Can you work these out from the model? Positions are in its coordinate system, mm. Face numbers are marked on the shaded views. A direction names the side the tool comes from. Coordinates: 2 decimals unless noted, no trailing zeros. Order: outer loops, then holes, each group sorted by start corner. A loop starts at its lowest first (then second) coordinate and runs counter-clockwise, first axis right, second up. Notation, with made-up numbers: (27.25, -7.75) -> (66.25, -7.75) arc R10 cw to (66.25, -0.75) -> close; hole circle Ø9 at (11.5, 70). An arc over 180 degrees is marked (long way). Return JSON: item names as keys, results as strings. Group by question number.
1) If we section it at B-B, the plane z = -7.5: Please give me the cut outline in (x, y).
2) Thinking about a two-plate mould opening in Z: for the marked faces 3, 4 and 5, which applies, +Z half, -Z half, draft (parallel to the pull), parting line (faces both ways), or undercut?
3) If I drill on probe 1 along Z at (x, y) = (0.5, -4); probe 2 along Z at (x, y) = (6.5, -11.5); probe 3 along Z at (x, y) = (-8.89, -7) (3 decimals), over which ranges is the centre line in solid material (lowest first)? Write a range as from..to.
4) For pin 1 (6.5 mm diameter, centred on y = -11.5, z = -25.5, fed in from +X); pin 2 (5 mm diameter, centred on x = 10, z = -53, fed in from +Y); pin 3 (9 mm diameter, centred on y = -11, z = -28.5, fed in from -X), each with a flat end and sliding along its axis, tell me the tip position at first contact or that it passes through.
5) If we section it at A-A, the plane z = -66.04: Please give me the cut outline in (x, y) (3 decimals).
6) If we section it at C-C, the plane x = 0: Please give me the cut outline in (y, z), then the cut area to 3 significant figures.
7) If we section it at D-D, the plane y = -3.5: State how many separate pieces and enclosed holes the cut face has, then the cut area to 3 significant figures.
8) For the marked faces 1 and 2, which set-ups out of +Z, -Z, +X, -X, +Y, -Y let a thin tool reach every point of the face, with its end or its side?
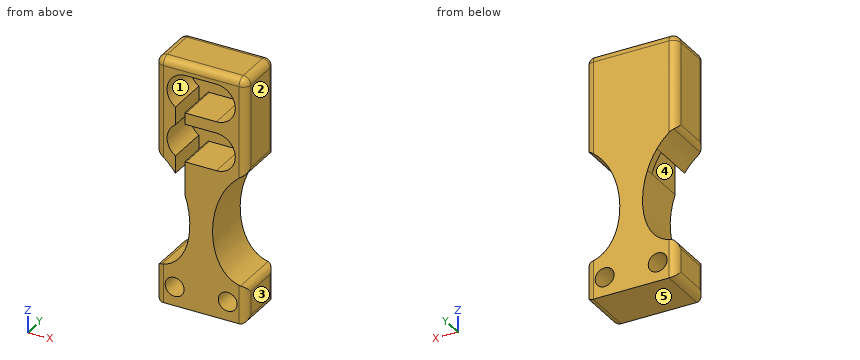
from build123d import *

# Parameters (mm, degrees)
F0_R     = 3.175
F1_DEPTH = 16.51
F2_DEPTH = 2.54
F3_R     = 2.54


# Not quite as in the source:
# - a feature names something its author has since deleted; it is built from what else it names


with BuildPart() as f1:
    # F0 (on Front) → F1 (new body)
    with BuildSketch(Plane.XZ):
        with BuildLine():
            Line((15.24, 10.16), (0, 10.16))
            Line((0, 10.16), (-15.24, 10.16))
            Line((-15.24, 10.16), (-15.24, -21.59))
            add(Edge.make_bspline(
                [(-15.24, -21.59), (-12.5713715272, -23.0241692542), (-10.3700381938, -25.1273333514), (-8.636, -27.620696738)],
                knots=[0, 0, 0, 0, 6.6715711821, 6.6715711821, 6.6715711821, 6.6715711821], degree=3))
            Line((-8.636, -27.620696738), (-8.636, -21.770928055))
            ThreePointArc((-8.636, -21.770928055), (-11.43, -16.51), (-8.636, -11.249071945))
            Line((-8.636, -11.249071945), (-8.636, -5.260928055))
            ThreePointArc((-8.636, -5.260928055), (-11.1516304709, 1.8595169871), (-5.08, 6.35))
            Line((-5.08, 6.35), (5.08, 6.35))
            ThreePointArc((5.08, 6.35), (9.5701280605, 4.4901280605), (11.43, 0))
            ThreePointArc((11.43, 0), (9.5701280605, -4.4901280605), (5.08, -6.35))
            Line((5.08, -6.35), (-5.08, -6.35))
            ThreePointArc((-5.08, -6.35), (-5.2705858603, -6.3471392792), (-5.461, -6.3385596944))
            Line((-5.461, -6.3385596944), (-5.461, -10.1714403056))
            ThreePointArc((-5.461, -10.1714403056), (-5.2705858603, -10.1628607208), (-5.08, -10.16))
            Line((-5.08, -10.16), (5.08, -10.16))
            ThreePointArc((5.08, -10.16), (9.5701280605, -12.0198719395), (11.43, -16.51))
            ThreePointArc((11.43, -16.51), (9.5701280605, -21.0001280605), (5.08, -22.86))
            Line((5.08, -22.86), (-5.08, -22.86))
            ThreePointArc((-5.08, -22.86), (-5.2705858603, -22.8571392792), (-5.461, -22.8485596944))
            Line((-5.461, -22.8485596944), (-5.461, -33.9487214282))
            add(Edge.make_bspline(
                [(-5.461, -33.9487214282), (-1.4642877536, -45.4909328609), (-4.7239544203, -59.7580237479), (-15.24, -59.69)],
                knots=[11.8098860506, 11.8098860506, 11.8098860506, 11.8098860506, 38.1, 38.1, 38.1, 38.1], degree=3))
            Line((-15.24, -59.69), (-15.24, -72.39))
            Line((-15.24, -72.39), (15.24, -72.39))
            Line((15.24, -72.39), (15.24, -59.69))
            add(Edge.make_bspline(
                [(15.24, -21.59), (0, -29.7802519053), (0, -59.7885809647), (15.24, -59.69)],
                knots=[0, 0, 0, 0, 38.1, 38.1, 38.1, 38.1], degree=3))
            Line((15.24, -21.59), (15.24, 10.16))
        make_face()
        with Locations((-8.89, -66.04)):
            Circle(F0_R, mode=Mode.SUBTRACT)
        with Locations((8.89, -66.04)):
            Circle(F0_R, mode=Mode.SUBTRACT)
    extrude(amount=F1_DEPTH)

    # F0 (on Front) → F2 (join)
    with BuildSketch(Plane.XZ):
        with BuildLine():
            ThreePointArc((-5.08, 6.35), (-11.1516304709, 1.8595169871), (-8.636, -5.260928055))
            ThreePointArc((-8.636, -5.260928055), (-7.1209102718, -6.0130845048), (-5.461, -6.3385596944))
            ThreePointArc((-5.461, -6.3385596944), (-5.2705858603, -6.3471392792), (-5.08, -6.35))
            ThreePointArc((-5.08, -6.35), (-2.2401936686, -5.6796126628), (0, -3.81))
            ThreePointArc((0, -3.81), (-1.27, 0), (0, 3.81))
            ThreePointArc((0, 3.81), (-2.2401936686, 5.6796126628), (-5.08, 6.35))
        make_face()
        with BuildLine():
            ThreePointArc((5.08, 6.35), (2.2401936686, 5.6796126628), (0, 3.81))
            ThreePointArc((0, 3.81), (0.9441389426, 2.0080463142), (1.27, 0))
            ThreePointArc((1.27, 0), (0.9441389426, -2.0080463142), (0, -3.81))
            ThreePointArc((0, -3.81), (2.2401936686, -5.6796126628), (5.08, -6.35))
            ThreePointArc((5.08, -6.35), (9.5701280605, -4.4901280605), (11.43, 0))
            ThreePointArc((11.43, 0), (9.5701280605, 4.4901280605), (5.08, 6.35))
        make_face()
        with BuildLine():
            Line((5.08, 6.35), (-5.08, 6.35))
            ThreePointArc((-5.08, 6.35), (-2.2401936686, 5.6796126628), (0, 3.81))
            ThreePointArc((0, 3.81), (2.2401936686, 5.6796126628), (5.08, 6.35))
        make_face()
        with BuildLine():
            ThreePointArc((1.27, 0), (0.9441389426, 2.0080463142), (0, 3.81))
            ThreePointArc((0, 3.81), (-1.27, 0), (0, -3.81))
            ThreePointArc((0, -3.81), (0.9441389426, -2.0080463142), (1.27, 0))
        make_face()
        with BuildLine():
            ThreePointArc((0, -3.81), (-2.2401936686, -5.6796126628), (-5.08, -6.35))
            Line((-5.08, -6.35), (5.08, -6.35))
            ThreePointArc((5.08, -6.35), (2.2401936686, -5.6796126628), (0, -3.81))
        make_face()
        with BuildLine():
            Line((-5.461, -22.5981636269), (-5.461, -22.8485596944))
            ThreePointArc((-5.461, -22.8485596944), (-5.2705858603, -22.8571392792), (-5.08, -22.86))
            ThreePointArc((-5.08, -22.86), (-2.2401936686, -22.1896126628), (0, -20.32))
            ThreePointArc((0, -20.32), (-1.27, -16.51), (0, -12.7))
            ThreePointArc((0, -12.7), (-2.2401936686, -10.8303873372), (-5.08, -10.16))
            ThreePointArc((-5.08, -10.16), (-5.2705858603, -10.1628607208), (-5.461, -10.1714403056))
            Line((-5.461, -10.1714403056), (-5.461, -22.5981636269))
        make_face()
        with BuildLine():
            ThreePointArc((0, -12.7), (-1.27, -16.51), (0, -20.32))
            ThreePointArc((0, -20.32), (0.9441389426, -18.5180463142), (1.27, -16.51))
            ThreePointArc((1.27, -16.51), (0.9441389426, -14.5019536858), (0, -12.7))
        make_face()
        with BuildLine():
            Line((5.08, -10.16), (-5.08, -10.16))
            ThreePointArc((-5.08, -10.16), (-2.2401936686, -10.8303873372), (0, -12.7))
            ThreePointArc((0, -12.7), (2.2401936686, -10.8303873372), (5.08, -10.16))
        make_face()
        with BuildLine():
            ThreePointArc((1.27, -16.51), (0.9441389426, -18.5180463142), (0, -20.32))
            ThreePointArc((0, -20.32), (2.2401936686, -22.1896126628), (5.08, -22.86))
            ThreePointArc((5.08, -22.86), (9.5701280605, -21.0001280605), (11.43, -16.51))
            ThreePointArc((11.43, -16.51), (9.5701280605, -12.0198719395), (5.08, -10.16))
            ThreePointArc((5.08, -10.16), (2.2401936686, -10.8303873372), (0, -12.7))
            ThreePointArc((0, -12.7), (0.9441389426, -14.5019536858), (1.27, -16.51))
        make_face()
        with BuildLine():
            ThreePointArc((0, -20.32), (-2.2401936686, -22.1896126628), (-5.08, -22.86))
            Line((-5.08, -22.86), (5.08, -22.86))
            ThreePointArc((5.08, -22.86), (2.2401936686, -22.1896126628), (0, -20.32))
        make_face()
        with BuildLine():
            Line((-8.636, -21.770928055), (-8.636, -27.620696738))
            add(Edge.make_bspline(
                [(-8.636, -27.620696738), (-7.3004773786, -29.5410369116), (-6.2421440453, -31.6928347959), (-5.461, -33.9487214282)],
                knots=[6.6715711821, 6.6715711821, 6.6715711821, 6.6715711821, 11.8098860506, 11.8098860506, 11.8098860506, 11.8098860506], degree=3))
            Line((-5.461, -33.9487214282), (-5.461, -22.8485596944))
            ThreePointArc((-5.461, -22.8485596944), (-7.1209102718, -22.5230845048), (-8.636, -21.770928055))
        make_face()
        with BuildLine():
            Line((-8.636, -5.260928055), (-8.636, -11.249071945))
            ThreePointArc((-8.636, -11.249071945), (-7.1209102718, -10.4969154952), (-5.461, -10.1714403056))
            Line((-5.461, -10.1714403056), (-5.461, -6.3385596944))
            ThreePointArc((-5.461, -6.3385596944), (-7.1209102718, -6.0130845048), (-8.636, -5.260928055))
        make_face()
        with BuildLine():
            ThreePointArc((-8.636, -11.249071945), (-11.43, -16.51), (-8.636, -21.770928055))
            ThreePointArc((-8.636, -21.770928055), (-7.1209102718, -22.5230845048), (-5.461, -22.8485596944))
            Line((-5.461, -22.8485596944), (-5.461, -22.5981636269))
            Line((-5.461, -22.5981636269), (-5.461, -10.1714403056))
            ThreePointArc((-5.461, -10.1714403056), (-7.1209102718, -10.4969154952), (-8.636, -11.249071945))
        make_face()
    extrude(amount=F2_DEPTH)

    # F3
    f3_edges = [f1.edges().sort_by_distance(p)[0] for p in [
        (15.24, -8.255, 10.16),
        (0, -16.51, 10.16),
        (-15.24, -8.255, 10.16),
        (0, 0, 10.16),
        (15.24, -8.255, -21.59),
        (15.24, 0, -5.715),
        (15.24, -16.51, -5.715),
        (-15.24, -8.255, -21.59),
        (-15.24, 0, -5.715),
        (-15.24, -16.51, -5.715),
        (15.24, -8.255, -72.39),
        (15.24, -8.255, -59.69),
        (15.24, 0, -66.04),
        (15.24, -16.51, -66.04),
        (-15.24, -8.255, -59.69),
        (-15.24, -8.255, -72.39),
        (-15.24, 0, -66.04),
        (-15.24, -16.51, -66.04),
    ]]
    fillet(f3_edges, radius=F3_R)


solid = f1.part
Result sheet:
{
 "1": {"outline": "(-15.24, -13.97) arc R2.54 ccw to (-12.7, -16.51) -> (-8.64, -16.51) -> (-8.64, -2.54) -> (-5.46, -2.54) -> (-5.46, -16.51) -> (12.7, -16.51) arc R2.54 ccw to (15.24, -13.97) -> (15.24, -2.54) arc R2.54 ccw to (12.7, 0) -> (-12.7, 0) arc R2.54 ccw to (-15.24, -2.54) -> close"},
 "2": {"face 3": "draft", "face 4": "undercut", "face 5": "-Z half"},
 "3": {"probe 1": "z = -72.39..-22.86, -10.16..-6.35, 6.35..10.16", "probe 2": "z = -72.39..-68.13, -63.95..-54.67, -31.37..-22.7, -10.32..-6.19, 6.19..10.16", "probe 3": "z = -72.39..-69.215, -62.865..-57.471, -27.263..-21.59, -11.43..-5.08, 5.08..10.16"},
 "4": {"pin 1": "stops at x = 14.12", "pin 2": "passes through", "pin 3": "stops at x = -11.82"},
 "5": {"outline": "(-15.24, -13.97) arc R2.54 ccw to (-12.7, -16.51) -> (-12.065, -16.51) -> (-12.065, 0) -> (-12.7, 0) arc R2.54 ccw to (-15.24, -2.54) -> close; (-5.715, -16.51) -> (5.715, -16.51) -> (5.715, 0) -> (-5.715, 0) -> close; (12.065, -16.51) -> (12.7, -16.51) arc R2.54 ccw to (15.24, -13.97) -> (15.24, -2.54) arc R2.54 ccw to (12.7, 0) -> (12.065, 0) -> close"},
 "6": {"outline": "(-16.51, -72.39) -> (0, -72.39) -> (0, 7.62) arc R2.54 ccw to (-2.54, 10.16) -> (-13.97, 10.16) arc R2.54 ccw to (-16.51, 7.62) -> (-16.51, 6.35) -> (-2.54, 6.35) -> (-2.54, -6.35) -> (-16.51, -6.35) -> (-16.51, -10.16) -> (-2.54, -10.16) -> (-2.54, -22.86) -> (-16.51, -22.86) -> close", "area": "1,010 mm2"},
 "7": {"separate pieces": "1", "enclosed holes": "2", "area": "1,230 mm2"},
 "8": {"face 1": "-Y", "face 2": "+Z, -Z, +X, +Y, -Y"}
}
